Could you check a few things on this model? Use its own coordinates, in mm. Face numbers are marked on the shaded views. Coordinates: 2 decimals unless noted, no trailing zeros. Order: outer loops, then holes, each group sorted by start corner. A loop starts at its lowest first (then second) coordinate and runs counter-clockwise, first axis right, second up. Notation, with made-up numbers: (51.25, 80.25) - (61.25, 80.25) arc R21 ccw to (61.25, 118.25) - close; hole circle Ø3 at (33.5, -22.5). An arc over 180 degrees is marked (long way). One line per item, written item: value. Start each with the question number.
from build123d import *

# Parameters (mm, degrees)
SKETCH_W     = 1.2
SKETCH_H     = 5
PAD_DEPTH    = 10
SKETCH001_R  = 1.25
POCKET_DEPTH = 1.2
FILLET_R     = 2.49


with BuildPart() as part:
    # Sketch → Pad (new body)
    with BuildSketch(Plane.XY):
        Rectangle(SKETCH_W, SKETCH_H)
    extrude(amount=-PAD_DEPTH)

    # Sketch001 (on Face3 of Pad) → Pocket (cut)
    with BuildSketch(Plane.YZ.offset(0.6)):
        with Locations((0, -7.5)):
            Circle(SKETCH001_R)
    extrude(amount=-POCKET_DEPTH, mode=Mode.SUBTRACT)

    # Fillet
    fillet_edges = [part.edges().sort_by_distance(p)[0] for p in [
        (0, -2.5, -10),
        (0, 2.5, -10),
    ]]
    fillet(fillet_edges, radius=FILLET_R)


solid = part.part
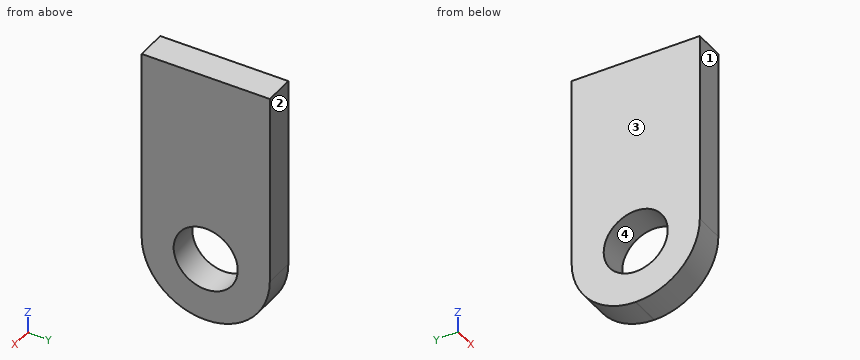
Q1. If I drill on L1, parallel to Z at x = 0.1, y = 0; L2, parallel to Z at x = -0.4, y = 0.8; L3, parallel to Y at x = -0.1, z = -8.5, over which ranges is the centre line in solid material (lowest first)?
Q2. I want a section at D-D on y = -1.35. Please give me the cut outline in (x, z), then the cut area to 3 significant figures.
Q3. We'd pull the mould along Y, two halves only. Please class the marked faces 1, 2, 3 and 4: +Y half, -Y half, draft (parallel to the pull), parting line (faces both ways), or undercut.
Q4. I want a section at A-A on y = 0.15. Please give me the cut outline in (x, z).
Q5. I want a section at C-C on y = -1.95. Please give me the cut outline in (x, z), then the cut area to 3 significant figures.
Values follow:
1. L1: z = -10 to -8.75, -6.25 to 0
1. L2: z = -9.87 to -8.46, -6.54 to 0
1. L3: y = -2.29 to -0.75, 0.75 to 2.29
2. outline: (-0.6, -9.61) - (0.6, -9.61) - (0.6, 0) - (-0.6, 0) - close
2. area: 11.5 mm^2
3. face 1: -Y half
3. face 2: +Y half
3. face 3: draft
3. face 4: undercut
4. outline: (-0.6, -10) - (0.6, -10) - (0.6, -8.74) - (-0.6, -8.74) - close; (-0.6, -6.26) - (0.6, -6.26) - (0.6, 0) - (-0.6, 0) - close
5. outline: (-0.6, -9.07) - (0.6, -9.07) - (0.6, 0) - (-0.6, 0) - close
5. area: 10.9 mm^2
